```python
from build123d import *
from build123d.topology import SkipClean

# Parameters (mm, degrees)
SKETCH1_R           = 21
BOSS_EXTRUDE1_DEPTH = 3.5
SKETCH4_R           = 10
CUT_EXTRUDE1_DEPTH  = 8.2
SKETCH11_R          = 1.5
CUT_EXTRUDE2_DEPTH  = 10
BOSS_EXTRUDE2_START = 11
BOSS_EXTRUDE2_DEPTH = 11
SKETCH14_R          = 1.5
CUT_EXTRUDE3_DEPTH  = 5
SKETCH16_R          = 3.55
BOSS_EXTRUDE3_DEPTH = 13.5
SKETCH17_R          = 4.5
BOSS_EXTRUDE4_DEPTH = 7


with BuildPart() as part:
    # Sketch1 → Boss-Extrude1 (new body)
    with BuildSketch(Plane.XY):
        Circle(SKETCH1_R)
    extrude(amount=BOSS_EXTRUDE1_DEPTH)

    # Sketch4 → Cut-Extrude1 (cut)
    with BuildSketch(Plane(origin=(0, 0, 0), x_dir=(-1, 0, 0), z_dir=(0, 0, -1))):
        Circle(SKETCH4_R)
    extrude(amount=-CUT_EXTRUDE1_DEPTH, mode=Mode.SUBTRACT)

    # Sketch11 → Cut-Extrude2 (cut)
    with BuildSketch(Plane(origin=(0, 0, 0), x_dir=(-1, 0, 0), z_dir=(0, 0, -1))):
        with Locations((0, 15)):
            Circle(SKETCH11_R)
        with Locations((12.990381057, -7.5)):
            Circle(SKETCH11_R)
        with Locations((-12.990381057, -7.5)):
            Circle(SKETCH11_R)
    extrude(amount=-CUT_EXTRUDE2_DEPTH, mode=Mode.SUBTRACT)

    # Sketch3 → Boss-Extrude2 (add)
    with SkipClean():  # the faces are left unmerged after this step: merging them gives an invalid solid
        with BuildSketch(Plane(origin=(0, 0, 0), x_dir=(-1, 0, 0), z_dir=(0, 0, -1)).offset(BOSS_EXTRUDE2_START)):
            with BuildLine():
                ThreePointArc((-3.021915591, -12.129221993), (-4.618435811, -16.247865366), (-7.4589705, -19.630684121))
                ThreePointArc((-7.4589705, -19.630684121), (0, -21), (7.4589705, -19.630684121))
                ThreePointArc((7.4589705, -19.630684121), (4.618435811, -16.247865366), (3.021915591, -12.129221993))
                ThreePointArc((3.021915591, -12.129221993), (0, -12.5), (-3.021915591, -12.129221993))
            make_face()
            with BuildLine():
                ThreePointArc((-20.730156393, 3.355684121), (-16.38028207, 4.124249945), (-12.01517217, 3.447555327))
                ThreePointArc((-12.01517217, 3.447555327), (-10.825317547, 6.25), (-8.993256579, 8.681666667))
                ThreePointArc((-8.993256579, 8.681666667), (-11.761846259, 12.123615422), (-13.271185893, 16.275))
                ThreePointArc((-13.271185893, 16.275), (-18.186533479, 10.5), (-20.730156393, 3.355684121))
            make_face()
            with BuildLine():
                ThreePointArc((8.993256579, 8.681666667), (10.825317547, 6.25), (12.01517217, 3.447555327))
                ThreePointArc((12.01517217, 3.447555327), (16.38028207, 4.124249945), (20.730156393, 3.355684121))
                ThreePointArc((20.730156393, 3.355684121), (18.186533479, 10.5), (13.271185893, 16.275))
                ThreePointArc((13.271185893, 16.275), (11.761846259, 12.123615422), (8.993256579, 8.681666667))
            make_face()
        extrude(amount=-BOSS_EXTRUDE2_DEPTH)

    # Sketch14 → Cut-Extrude3 (cut)
    with SkipClean():  # the faces are left unmerged after this step: merging them gives an invalid solid
        with BuildSketch(Plane(origin=(0, 0, -11), x_dir=(-1, 0, 0), z_dir=(0, 0, -1))):
            with Locations((13.856406461, 8)):
                Circle(SKETCH14_R)
            with Locations((0, -16)):
                Circle(SKETCH14_R)
            with Locations((-13.856406461, 8)):
                Circle(SKETCH14_R)
        extrude(amount=-CUT_EXTRUDE3_DEPTH, mode=Mode.SUBTRACT)

    # Sketch16 → Boss-Extrude3 (add)
    with SkipClean():  # the faces are left unmerged after this step: merging them gives an invalid solid
        with BuildSketch(Plane.XY.offset(3.5)):
            with Locations((0, 15)):
                Circle(SKETCH16_R)
            with Locations((12.990381057, -7.5)):
                Circle(SKETCH16_R)
            with Locations((-12.990381057, -7.5)):
                Circle(SKETCH16_R)
        extrude(amount=-BOSS_EXTRUDE3_DEPTH)

    # Sketch17 → Boss-Extrude4 (add)
    with SkipClean():  # the faces are left unmerged after this step: merging them gives an invalid solid
        with BuildSketch(Plane(origin=(0, 0, 0), x_dir=(-1, 0, 0), z_dir=(0, 0, -1))):
            with Locations(Location((0, 15, 0), (0, 0, 180))):
                Circle(SKETCH17_R)
            with Locations(Location((12.990381057, -7.5, 0), (0, 0, 180))):
                Circle(SKETCH17_R)
            with Locations(Location((-12.990381057, -7.5, 0), (0, 0, 180))):
                Circle(SKETCH17_R)
        extrude(amount=BOSS_EXTRUDE4_DEPTH)


solid = part.part
```
Check sheet for the modelled part. Datum: model origin and axes. Units: mm. A direction names the side the tool comes from. Round coordinates to 2 decimals unless told otherwise and drop trailing zeros. Order: outer loops, then holes, each group sorted by start corner. A loop starts at its lowest first (then second) coordinate and runs counter-clockwise, first axis right, second up.
1) Scan lines: line 1 (Y direction, x = -0.5, z = -9.75); line 2 (X direction, y = 12, z = -8); line 3 (Y direction, x = 0, z = 1.95). Record each from-to range of solid material in increasing order.
2) Go/stop test with flat-tipped pins: pin 1 Ø5.5 at (x, y) = (11.5, -9) entering from -Z; pin 2 Ø1.8 at (x, y) = (0, -16) entering from -Z; pin 3 Ø5 at (y, z) = (15.5, -7.5) entering from -X. Record where each tip stops, or that it passes through.
3) Section check D-D (y = 8). Record the boundary of the cut face in (x, z).
4) Mould release check, pull along Y, two halves, no side actions. Record for faces 4 (the flat face through (9, 5, 3.5)), 5 (the flat face through (-12.7, -11.2, -7)), 6 (the cylindrical face through (-11.792, 12.178, -5.577)): +Y half, -Y half, draft (parallel to the pull), parting line (faces both ways), or undercut.
5) Section check C-C (z = -0.75). Record the boundary of the cut face in (x, y) (3 decimals).
6) Section check A-A (z = -9.25). Give the number of separate pieces and of enclosed holes in the cut face, and give its area (3 significant figures).
7) Section check B-B (x = 0). Record the boundary of the cut face in (y, z), and give its area (3 significant figures).
8) Tool access check on faces 1 (the flat face through (-14, 8, -6)), 2 (the cylindrical face through (11.73, 12.07, -5.58)), 3 (the cylindrical face through (4.587, -16.194, -5.577)). Record the directions out of +Z, -Z, +X, -X, +Y, -Y that give a thin tool (end or side, any length) a straight path to the whole face; none if there is none.
Result:
1. line 1: y = -20.99 to -17.41, -14.59 to -12.49, 11.49 to 18.51
1. line 2: x = -17.23 to -11.69, -1.9 to 1.9, 11.69 to 17.23
1. line 3: y = -21 to -10, 10 to 21
2. pin 1: stops at z = -10
2. pin 2: stops at z = -6
2. pin 3: stops at x = -16.49
3. outline: (-19.42, -11) - (-15.36, -11) - (-15.36, -6) - (-12.36, -6) - (-12.36, -11) - (-9.6, -11) - (-9.6, 0) - (-6, 0) - (-6, 3.5) - (-19.42, 3.5) - close; (6, 0) - (9.6, 0) - (9.6, -11) - (12.36, -11) - (12.36, -6) - (15.36, -6) - (15.36, -11) - (19.42, -11) - (19.42, 3.5) - (6, 3.5) - close
4. face 4: draft
4. face 5: undercut
4. face 6: +Y half
5. outline: (-20.73, 3.356) arc R13.5 cw to (-12.015, 3.448) arc R12.5 cw to (-8.993, 8.682) arc R13.5 cw to (-13.271, 16.275) arc R21 ccw to start; circle Ø9 at (-12.99, -7.5); (-7.459, -19.631) arc R21 ccw to (7.459, -19.631) arc R13.5 cw to (3.022, -12.129) arc R12.5 cw to (-3.022, -12.129) arc R13.5 cw to start; circle Ø9 at (0, 15); circle Ø9 at (12.99, -7.5); (8.993, 8.682) arc R12.5 cw to (12.015, 3.448) arc R13.5 cw to (20.73, 3.356) arc R21 ccw to (13.271, 16.275) arc R13.5 cw to start
6. separate pieces: 6
6. enclosed holes: 3
6. area: 345 mm2
7. outline: (-21, -11) - (-17.5, -11) - (-17.5, -6) - (-14.5, -6) - (-14.5, -11) - (-12.5, -11) - (-12.5, 0) - (-10, 0) - (-10, 3.5) - (-21, 3.5) - close; (10, 0) - (10.5, 0) - (10.5, -7) - (11.45, -7) - (11.45, -10) - (18.55, -10) - (18.55, -7) - (19.5, -7) - (19.5, 0) - (21, 0) - (21, 3.5) - (10, 3.5) - close
7. area: 240 mm2
8. face 1: -Z
8. face 2: -Z, +Y
8. face 3: -Z, +X
